For this review, take the finished solid that the model builds, in its own axes (mm). A direction names the side the tool comes from. Coordinates: 2 decimals unless noted, no trailing zeros. Write each loop counter-clockwise with the first axis right and the second up, starting at its lowest first coordinate (ties: lowest second). Pieces come first, ordered by that corner, then holes. Notation, with made-up numbers: (55.5, 2.5) - (66.5, 2.5) arc R22 cw to (66.5, 16.5) - close; hole circle Ø6 at (-29.5, 73.5). An arc over 180 degrees is marked (long way). Write each question's results on one line, items separated by ' | '.
from build123d import *

# Parameters (mm, degrees)
F1_DEPTH = 64
F3_DEPTH = 370
F6_DEPTH = 500
F8_R     = 15.9
F9_DEPTH = 600


# Not quite as in the source:
# - a feature names something its author has since deleted; it is built from what else it names


with BuildPart() as f1:
    # F0 (on Right) → F1 (new body, symmetric)
    with BuildSketch(Plane.YZ):
        with BuildLine():
            Line((380, 0), (0, 0))
            ThreePointArc((0, 0), (-20.7082948253, 4.5909184352), (-37.5361777128, 17.5034071254))
            Line((-37.5361777128, 17.5034071254), (-121, 116.9717171877))
            Line((-121, 116.9717171877), (-187.1849916482, 195.8479187603))
            Line((-187.1849916482, 195.8479187603), (-187.8376952929, 195.0700568469))
            Line((-187.8376952929, 195.0700568469), (-128.3694552412, 124.1985681201))
            Line((-128.3694552412, 124.1985681201), (-38.3022221559, 16.8606195157))
            ThreePointArc((-38.3022221559, 16.8606195157), (-21.130913087, 3.6846106482), (0, -1))
            Line((0, -1), (380, -1))
            ThreePointArc((380, -1), (400.9643426533, 1.7600080706), (420.5, 9.8519422935))
            Line((420.5, 9.8519422935), (446.4807621135, 24.8519422935))
            Line((446.4807621135, 24.8519422935), (445.9807621135, 25.7179676972))
            Line((445.9807621135, 25.7179676972), (420, 10.7179676972))
            ThreePointArc((420, 10.7179676972), (400.7055236082, 2.7259338969), (380, 0))
        make_face()
    extrude(amount=F1_DEPTH, both=True)

    # F2 (on Front) → F3 (join)
    with BuildSketch(Plane.XZ):
        with BuildLine():
            ThreePointArc((65.041889066, -11.9088465181), (69.9771681886, -5.4770655435), (64, 0))
            Line((64, 0), (-64, 0))
            ThreePointArc((-64, 0), (-69.9771681886, -5.4770655435), (-65.041889066, -11.9088465181))
            Line((-65.041889066, -11.9088465181), (-30.1606090351, -18.0593573092))
            Line((-30.1606090351, -18.0593573092), (-29.9869608574, -17.0745495562))
            Line((-29.9869608574, -17.0745495562), (-64.8682408883, -10.9240387651))
            ThreePointArc((-64.8682408883, -10.9240387651), (-68.9809734905, -5.5642212863), (-64, -1))
            Line((-64, -1), (64, -1))
            ThreePointArc((64, -1), (68.9809734905, -5.5642212863), (64.8682408883, -10.9240387651))
            Line((64.8682408883, -10.9240387651), (29.9869608574, -17.0745495562))
            Line((29.9869608574, -17.0745495562), (30.1606090351, -18.0593573092))
            Line((30.1606090351, -18.0593573092), (65.041889066, -11.9088465181))
        make_face()
    extrude(amount=-F3_DEPTH)

    # F5 (on offset) → F6 (cut)
    with BuildSketch(Plane.XY.offset(400)):
        with BuildLine():
            Line((-25, 446.4807621135), (-25, 385))
            ThreePointArc((-25, 385), (0, 360), (25, 385))
            Line((25, 385), (25, 446.4807621135))
            Line((25, 446.4807621135), (-25, 446.4807621135))
        make_face()
    extrude(amount=-F6_DEPTH, mode=Mode.SUBTRACT)

    # F8 (on offset) → F9 (cut)
    with BuildSketch(Plane(origin=(0, 369.6138337955, 310.1428316158), x_dir=(-1, 0, 0), z_dir=(0, 0.7660444431, 0.6427876097))):
        with Locations((0, 167.3828347258)):
            Circle(F8_R)
        with BuildLine():
            ThreePointArc((-40, 167.3828347258), (0, 207.3828347258), (40, 167.3828347258))
            Line((40, 167.3828347258), (40, 127.3828347258))
            ThreePointArc((40, 127.3828347258), (46.052321998, 62.5708246837), (64, 0))
            Line((64, 0), (64, 37.5361777128))
            Line((64, 37.5361777128), (64, 270.3484032135))
            Line((64, 270.3484032135), (-64, 270.3484032135))
            Line((-64, 270.3484032135), (-64, 37.5361777128))
            Line((-64, 37.5361777128), (-64, 0))
            ThreePointArc((-64, 0), (-46.052321998, 62.5708246837), (-40, 127.3828347258))
            Line((-40, 127.3828347258), (-40, 167.3828347258))
        make_face()
    extrude(amount=-F9_DEPTH, mode=Mode.SUBTRACT)


solid = f1.part
Q1. Take a section at B-B on y = 401.5. State the section outline as (x, z) points.
Results found:
outline: (-64, 1.91) - (-25, 1.91) - (-25, 2.94) - (-64, 2.94) - close; (25, 1.91) - (64, 1.91) - (64, 2.94) - (25, 2.94) - close
Q2. For faces 5 (the face through (-47.183, 182.41, -14.042)), 6 (the face through (44.77, 433.31, 17.25)), 7 (the face through (44.524, 400.989, 2.802)), 8 (the face through (64, 410.9, 5.5)), 9 (the face through (25, 416, 8)), list the 3-axis set-ups (+Z, -Z, +X, -X, +Y, -Y) from which the entire face can be reached by the end or side of a thin tool; tool diameter is ignored.
Results found:
face 5: +Y, -Y | face 6: -Z, +X, -X, +Y | face 7: +Z, +X, -X | face 8: +Z, -Z, +X, +Y | face 9: +Z, -Z, +Y
Q3. Take a section at A-A on x = 0. State the section outline as (y, z) points, plus the area to 3 significant figures.
Results found:
outline: (-147.48, 146.97) - (-131.99, 128.51) - (-131.22, 129.15) - (-146.71, 147.61) - close; (-111.55, 104.15) - (-38.3, 16.86) arc R50 ccw to (0, -1) - (360, -1) - (360, 0) - (0, 0) arc R49 cw to (-37.54, 17.5) - (-110.78, 104.79) - close | area: 541 mm2
Q4. Mouldability with a two-part tool opening along X and no side actions: class faces 1 (the face through (54, 0, -13)), 2 (the face through (40, -108, 101)), 3 (the face through (0.88, -147.08, 147.29)), 4 (the face through (-69, 182, -6)) as pulls with the +X half, pulls with the -X half, needs draft (parallel to the pull), parting line crosses it, or undercut.
Results found:
face 1: needs draft | face 2: pulls with the +X half | face 3: parting line crosses it | face 4: undercut
Q5. For pin 1 (10 mm diameter, centred on x = -11.5, y = -52.5, fed in from -Z); pin 2 (1.5 mm diameter, centred on x = -48, y = 308.5, fed in from -Z); pin 3 (1.1 mm diameter, centred on y = -1, z = -0.5, fed in from -X); pin 4 (9 mm diameter, centred on x = -50.5, z = -8, fed in from -Y), all flat-tipped, find the tip position at first contact; note any pin that passes through.
Results found:
pin 1: z = 27.82 | pin 2: z = -15.05 | pin 3: x = -64 | pin 4: through
Q6. Take a section at C-C on y = 102. State the section outline as (x, z) points, plus the area to 3 significant figures.
Results found:
outline: (-65.04, -11.91) - (-30.16, -18.06) - (-29.99, -17.07) - (-64.87, -10.92) arc R5 cw to (-64, -1) - (64, -1) arc R5 cw to (64.87, -10.92) - (29.99, -17.07) - (30.16, -18.06) - (65.04, -11.91) arc R6 ccw to (64, 0) - (-64, 0) arc R6 ccw to start | area: 231 mm2
Q7. Take a section at D-D on z = 98. State the section outline as (x, y) points.
Results found:
outline: (-40, -106.39) - (40, -106.39) - (40, -105.08) - (-40, -105.08) - close
Q8. Wall thickness on line 1 along Z through (x, y) = (-15.5, 10.5); line 2 along Z through (x, y) = (-36, 287.5); line 3 along Z through (x, y) = (60.5, 122.5): over which ranges is each line inside the solid? List them lowest first. Write a range as from..to.
Results found:
line 1: -1..0 | line 2: -17.03..-16.01, -1..0 | line 3: -12.71..-11.69, -1..0
